Verification items for this drawing (mm, ordinates from the low corner). A direction names the side the tool comes from. Round coordinates to 2 decimals unless told otherwise and drop trailing zeros. Write each loop counter-clockwise with the first axis right and the second up, starting at its lowest first coordinate (ties: lowest second). Pieces come first, ordered by that corner, then holes.
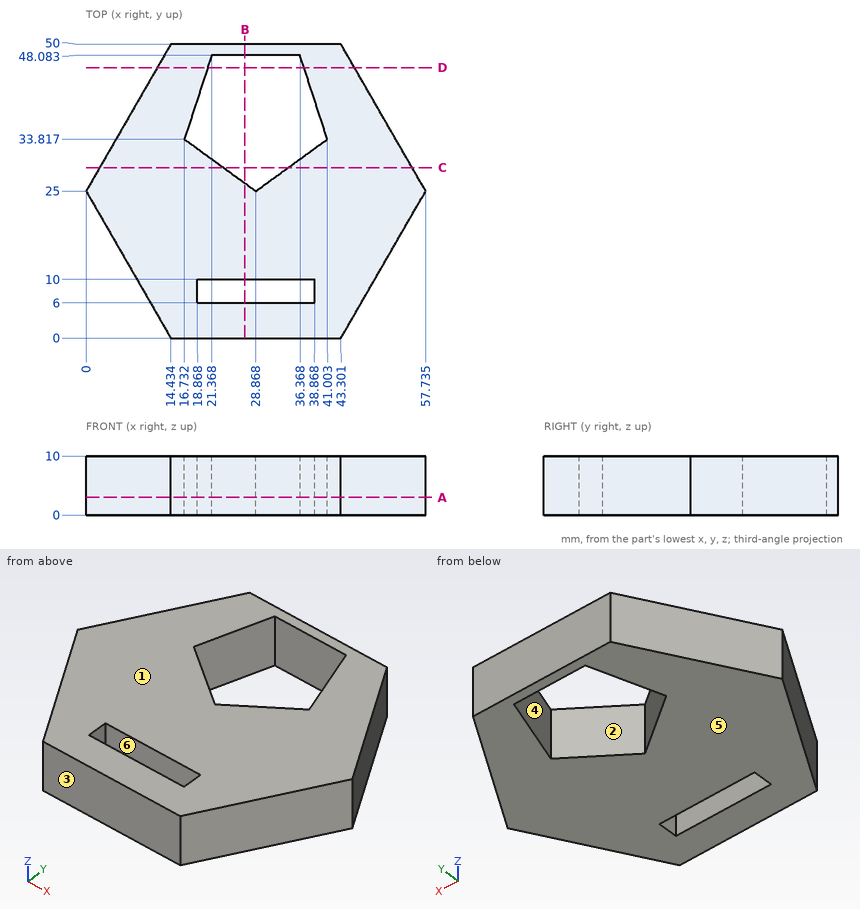
1. Release check for a two-part mould opening along Y. For the marked faces 3, 4, 5 and 6 record: +Y half, -Y half, draft (parallel to the pull), parting line (faces both ways), or undercut.
2. Scan lines: line 1 along Y through (x, z) = (30, 4) (1 decimal); line 2 along Y through (x, z) = (22.5, 7) (1 decimal); line 3 along X through (y, z) = (31, 0.75) (1 decimal). Record each from-to range of solid material in increasing order.
3. Section check C-C (y = 29). Record the cut outline in (x, z) (1 decimal).
4. Access from +Z, -Z, +X, -X, +Y, -Y to the whole of each face (thin tool, end or side, straight path). Record for the marked faces 1 and 2.
5. Section check D-D (y = 46). Record the cut outline in (x, z) (1 decimal).
6. Section check B-B (x = 27). Record the cut outline in (y, z).
7. Depth check by flat-ended pin: pin 1 Ø2 at (y, z) = (8, 4) entering from -X; pin 2 Ø1.2 at (y, z) = (8, 6) entering from +X; pin 3 Ø1 at (y, z) = (10, 6) entering from +X. Enter the tip coordinate at first touch or a pass-through.
8. Section check A-A (z = 3). Record the cut outline in (x, y) (1 decimal).
Results below:
1. face 3: -Y half
1. face 4: undercut
1. face 5: draft
1. face 6: undercut
2. line 1: y = 0 to 6, 10 to 25.8, 48.1 to 50
2. line 2: y = 0 to 6, 10 to 29.6, 48.1 to 50
2. line 3: x = 3.5 to 20.6, 37.1 to 54.3
3. outline: (2.3, 0) - (23.4, 0) - (23.4, 10) - (2.3, 10) - close; (34.4, 0) - (55.4, 0) - (55.4, 10) - (34.4, 10) - close
4. face 1: +Z, +X, -X, +Y, -Y
4. face 2: +Z, -Z
5. outline: (12.1, 0) - (20.7, 0) - (20.7, 10) - (12.1, 10) - close; (37, 0) - (45.6, 0) - (45.6, 10) - (37, 10) - close
6. outline: (0, 0) - (6, 0) - (6, 10) - (0, 10) - close; (10, 0) - (26.36, 0) - (26.36, 10) - (10, 10) - close; (48.08, 0) - (50, 0) - (50, 10) - (48.08, 10) - close
7. pin 1: stops at x = 9.24
7. pin 2: stops at x = 48.27
7. pin 3: stops at x = 49.36
8. outline: (0, 25) - (14.4, 0) - (43.3, 0) - (57.7, 25) - (43.3, 50) - (14.4, 50) - close; hole (16.7, 33.8) - (28.9, 25) - (41, 33.8) - (36.4, 48.1) - (21.4, 48.1) - close; hole (18.9, 6) - (38.9, 6) - (38.9, 10) - (18.9, 10) - close
